Part print with two shaded views. Sizes in mm from the minimum x, y, z corner. Give positions to 0.01 mm unless a question says otherwise; leave off trailing zeros. Order: outer loops, then holes, each group sorted by start corner. A loop starts at its lowest first (then second) coordinate and runs counter-clockwise, first axis right, second up. Notation, with made-up numbers: M 22,-24.75 L 36,-24.75 A35 cw 36,13.25 Z; hole C 46,35.25 d9. An arc over 180 degrees is marked long. Return JSON: item names as keys, results as strings.
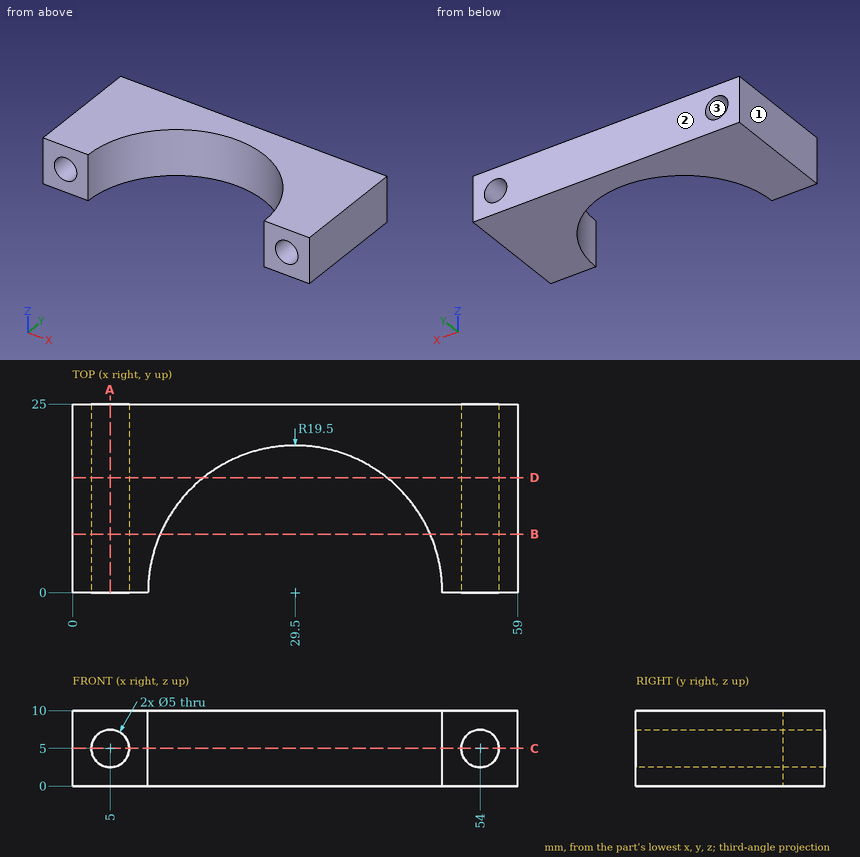
Q1. Band-saw the part on C-C (z = 5). Give the cut face in (x, y).
Established:
{"outline": "M 0,0 L 2.5,0 L 2.5,25 L 0,25 Z; M 7.5,0 L 10,0 A19.5 cw 49,0 L 51.5,0 L 51.5,25 L 7.5,25 Z; M 56.5,0 L 59,0 L 59,25 L 56.5,25 Z"}
Q2. Two-plate mould, pull along X, no slides. Class the marked faces 1, 2 and 3: +X half, -X half, draft (parallel to the pull), parting line (faces both ways), or undercut.
Established:
{"face 1": "-X half", "face 2": "draft", "face 3": "undercut"}
Q3. Band-saw the part on D-D (y = 15.25). Give the cut face in (x, z), then the cut area to 3 significant figures.
Established:
{"outline": "M 0,0 L 17.35,0 L 17.35,10 L 0,10 Z; M 41.65,0 L 59,0 L 59,10 L 41.65,10 Z; hole C 5,5 d5; hole C 54,5 d5", "area": "308 mm²"}
Q4. Band-saw the part on B-B (y = 7.75). Give the cut face in (x, z).
Established:
{"outline": "M 0,0 L 11.61,0 L 11.61,10 L 0,10 Z; M 47.39,0 L 59,0 L 59,10 L 47.39,10 Z; hole C 5,5 d5; hole C 54,5 d5"}
Q5. Band-saw the part on A-A (x = 5). Give the cut face in (y, z), then the cut area to 3 significant figures.
Established:
{"outline": "M 0,0 L 25,0 L 25,2.5 L 0,2.5 Z; M 0,7.5 L 25,7.5 L 25,10 L 0,10 Z", "area": "125 mm²"}
Q6. Probe line 1 along X through (y, z) = (21, 5.25); line 2 along Z through (x, y) = (54, 12.25); line 3 along X through (y, z) = (12, 5). List the from-to ranges inside material, lowest first.
Established:
{"line 1": "x = 0 to 2.51, 7.49 to 51.51, 56.49 to 59", "line 2": "z = 0 to 2.5, 7.5 to 10", "line 3": "x = 0 to 2.5, 7.5 to 14.13, 44.87 to 51.5, 56.5 to 59"}
Q7. Pin check, flat tips, straight feed: pin 1 (4 mm diameter, centred on x = 20.5, z = 7, fed in from -Y); pin 2 (10 mm diameter, centred on x = 24, y = 15.5, fed in from -Z). Stop position of each tip, or through.
Established:
{"pin 1": "stops at y = 16.1", "pin 2": "stops at z = 0"}
